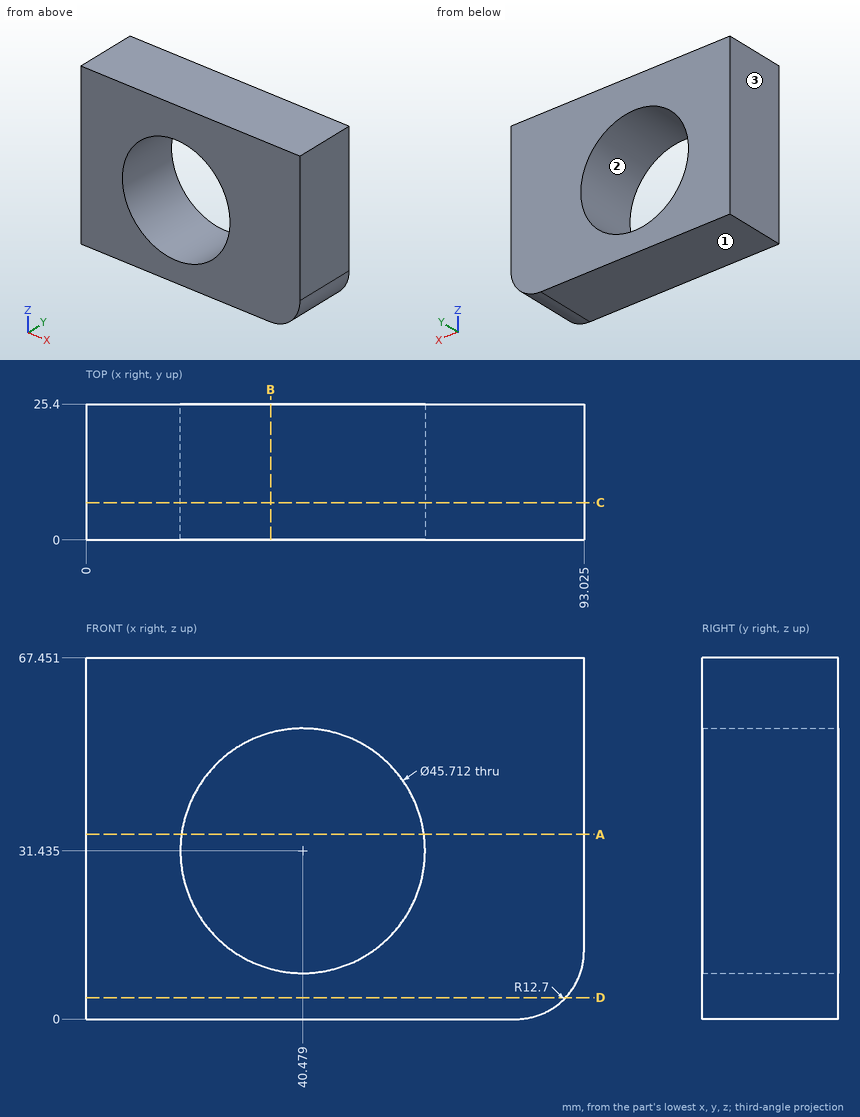
For this review, use the dimensioned drawing (mm, ordinates from the lowest corner) and the shaded views. Give positions to 0.01 mm unless a question says otherwise; leave off trailing zeros. Order: outer loops, then holes, each group sorted by start corner. A loop starts at its lowest first (then second) coordinate and runs counter-clockwise, first axis right, second up.
1) Take a section at A-A (z = 34.5). Give the boundary of the cut face in (x, y) (1 decimal), then the cut area to 3 significant figures.
2) Insertion check: pin 1 (5 mm diameter, centred on x = 42, z = 50, fed in from +Y). The pin has a flat end and moves straight along its axis. Give the tip position at first contact, or say it passes through.
3) Take a section at D-D (z = 4). Give the boundary of the cut face in (x, y).
4) The part is to be moulded in two halves that separate along Z. For the marked faces 1, 2 and 3, say which applies: released by +Z, released by -Z, zero draft, split by the parting line, or undercut.
5) Take a section at B-B (x = 34.5). Give the boundary of the cut face in (y, z) (1 decimal).
6) Take a section at C-C (y = 7). Give the boundary of the cut face in (x, z) (1 decimal), then the cut area to 3 significant figures.
7) Wall thickness on line 1 (X direction, y = 8.25, z = 45.5) (1 decimal); line 2 (X direction, y = 24.25, z = 18) (1 decimal); line 3 (Z direction, x = 51.5, y = 14): over which ranges is each line inside the solid? List them lowest first.
Derived:
1. outline: (0, 0) - (17.8, 0) - (17.8, 25.4) - (0, 25.4) - close; (63.1, 0) - (93, 0) - (93, 25.4) - (63.1, 25.4) - close
1. area: 1,210 mm2
2. pin 1: passes through
3. outline: (0, 0) - (89.58, 0) - (89.58, 25.4) - (0, 25.4) - close
4. face 1: released by -Z
4. face 2: undercut
4. face 3: zero draft
5. outline: (0, 0) - (25.4, 0) - (25.4, 9.4) - (0, 9.4) - close; (0, 53.5) - (25.4, 53.5) - (25.4, 67.5) - (0, 67.5) - close
6. outline: (0, 0) - (80.3, 0) arc R12.7 ccw to (93, 12.7) - (93, 67.5) - (0, 67.5) - close; hole circle Ø45.7 at (40.5, 31.4)
6. area: 4,600 mm2
7. line 1: x = 0 to 22.5, 58.5 to 93
7. line 2: x = 0 to 22, 59 to 93
7. line 3: z = 0 to 11.41, 51.46 to 67.45
